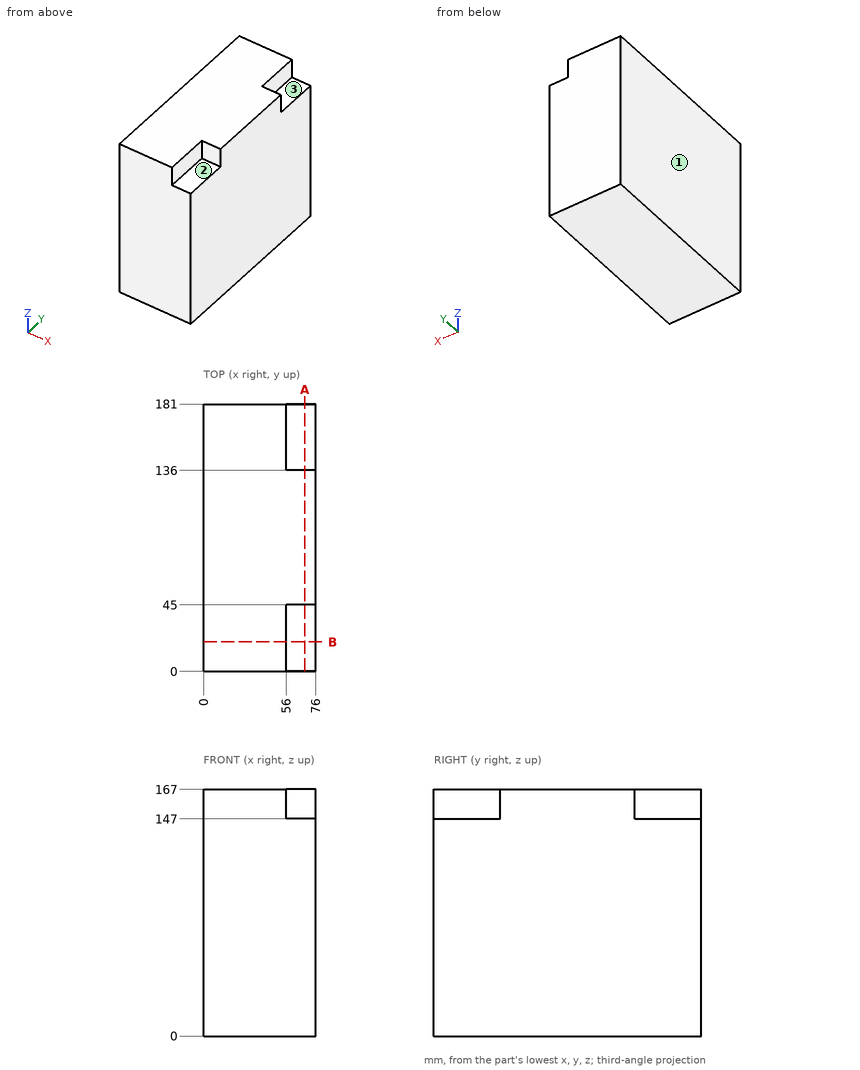
Answer from the drawing. Dimensions are ordinates in mm from the lowest x, y and z of the part. A direction names the side the tool comes from. Coordinates: 2 decimals unless noted, no trailing zeros. Loops run counter-clockwise (first coordinate to the right, second up) from the corner with the lowest first, then second, coordinate; pieces in that order, holes last.
Q1. Which of the six approach directions +Z, -Z, +X, -X, +Y, -Y give full straight-line access (tool end or side, diameter ignored) to the marked faces 1, 2 and 3?
Q2. The part is cut by section B-B on y = 20. Write down the section's boundary in (x, z).
Q3. The part is cut by section A-A on x = 68.5. Write down the section's boundary in (y, z).
Q4. Each of these flat-tipped pins is pushed along its axis until it touches: pin 1 Ø6 at (y, z) = (24, 153) entering from +X; pin 2 Ø3 at (x, y) = (62, 157) entering from +Z; pin 3 Ø10 at (x, z) = (68, 154) entering from -Y. Where does it stop, or does it pass through?
Q5. Consider probe 1 along Z at (x, y) = (60.5, 140). Determine where the line is inside the solid, lowest interval first.
Results below:
1. face 1: +Z, -Z, -X, +Y, -Y
1. face 2: +Z, +X, -Y
1. face 3: +Z, +X, +Y
2. outline: (0, 0) - (76, 0) - (76, 147) - (56, 147) - (56, 167) - (0, 167) - close
3. outline: (0, 0) - (181, 0) - (181, 147) - (136, 147) - (136, 167) - (45, 167) - (45, 147) - (0, 147) - close
4. pin 1: stops at x = 56
4. pin 2: stops at z = 147
4. pin 3: stops at y = 45
5. probe 1: z = 0 to 147
